from build123d import *

# Parameters (mm, degrees)
CROQUIS1_W                   = 75
CROQUIS1_H                   = 55
SALIENTE_EXTRUIR1_DEPTH      = 1.5
REDONDEO1_R                  = 3
TALADRO_DE_MARGEN_PARA_M31_D = 3.2
CROQUIS4_W                   = 14.87
CROQUIS4_H                   = 18.75
SALIENTE_EXTRUIR2_DEPTH      = 15.86
CROQUIS5_W                   = 30.45
CROQUIS5_H                   = 6.67
SALIENTE_EXTRUIR3_DEPTH      = 9.67
CROQUIS6_W                   = 15.19
CROQUIS6_H                   = 2.5
SALIENTE_EXTRUIR4_DEPTH      = 2.39
CROQUIS7_W                   = 0.67
CROQUIS7_H                   = 0.67
SALIENTE_EXTRUIR5_DEPTH      = 5.8


with BuildPart() as part:
    # Croquis1 → Saliente-Extruir1 (new body)
    with BuildSketch(Plane.XY):
        Rectangle(CROQUIS1_W, CROQUIS1_H)
    extrude(amount=SALIENTE_EXTRUIR1_DEPTH)

    # Redondeo1
    redondeo1_edges = [part.edges().sort_by_distance(p)[0] for p in [
        (-37.5, 27.5, 0.75),
        (37.5, 27.5, 0.75),
        (37.5, -27.5, 0.75),
        (-37.5, -27.5, 0.75),
    ]]
    fillet(redondeo1_edges, radius=REDONDEO1_R)

    # Taladro de margen para M31 (through all)
    with Locations(Plane.XY.offset(1.5)):
        with Locations((-34, 24), (-34, -24), (34, 24), (34, -24)):
            Hole(TALADRO_DE_MARGEN_PARA_M31_D / 2)

    # Croquis4 → Saliente-Extruir2 (add)
    with BuildSketch(Plane.XY.offset(1.5)):
        with Locations((-26.065, 4.905)):
            Rectangle(CROQUIS4_W, CROQUIS4_H)
        with Locations((-8.985, 4.905)):
            Rectangle(CROQUIS4_W, CROQUIS4_H)
        with Locations((8.985, 4.905)):
            Rectangle(CROQUIS4_W, CROQUIS4_H)
        with Locations((26.065, 4.905)):
            Rectangle(CROQUIS4_W, CROQUIS4_H)
    extrude(amount=SALIENTE_EXTRUIR2_DEPTH)

    # Croquis5 → Saliente-Extruir3 (add)
    with BuildSketch(Plane.XY.offset(1.5)):
        with Locations((-16.735, 19.265)):
            Rectangle(CROQUIS5_W, CROQUIS5_H)
        with Locations((16.735, 19.265)):
            Rectangle(CROQUIS5_W, CROQUIS5_H)
    extrude(amount=SALIENTE_EXTRUIR3_DEPTH)

    # Croquis6 → Saliente-Extruir4 (add)
    with BuildSketch(Plane.XY.offset(1.5)):
        with Locations((22.865, -22.54)):
            Rectangle(CROQUIS6_W, CROQUIS6_H)
    extrude(amount=SALIENTE_EXTRUIR4_DEPTH)

    # Croquis7 → Saliente-Extruir5 (add)
    with BuildSketch(Plane.XY.offset(3.89)):
        with Locations((16.465, -22.54)):
            Rectangle(CROQUIS7_W, CROQUIS7_H)
        with Locations((19.025, -22.54)):
            Rectangle(CROQUIS7_W, CROQUIS7_H)
        with Locations((21.585, -22.54)):
            Rectangle(CROQUIS7_W, CROQUIS7_H)
        with Locations((24.145, -22.54)):
            Rectangle(CROQUIS7_W, CROQUIS7_H)
        with Locations((26.705, -22.54)):
            Rectangle(CROQUIS7_W, CROQUIS7_H)
        with Locations((29.265, -22.54)):
            Rectangle(CROQUIS7_W, CROQUIS7_H)
    extrude(amount=SALIENTE_EXTRUIR5_DEPTH)


solid = part.part
CAD build for the part. Positions are in the model's coordinates, mm. A direction names the side the tool comes from. Round coordinates to 2 decimals unless told otherwise and drop trailing zeros. Write each loop counter-clockwise with the first axis right and the second up, starting at its lowest first coordinate (ties: lowest second). Pieces come first, ordered by that corner, then holes.
(1) 3-axis set-ups, long thin cutter, end or side, ignore diameter. For faces 4 (the face through (30.46, -23, 3)), 5 (the face through (-9, 14.28, 9)), 6 (the face through (33.5, 5, 9)), 7 (the face through (-1.51, 19, 6)), 8 (the face through (17, 22.6, 6)): which of +Z, -Z, +X, -X, +Y, -Y reach the whole face in a straight line?
(2) Mould opens along Y. For faces 1 (the face through (-26, 5, 17.36)), 2 (the face through (36.6, -26.64, 0.76)), 3 (the face through (-17, 15.93, 6)) say: pulls with the +Y half, pulls with the -Y half, needs draft (parallel to the pull), parting line crosses it, or undercut.
(3) Slice it at B-B, the plane z = 3. Write the cut outline in (x, y), and give its area (3 significant figures).
(4) Slice it at C-C, the plane y = 17. Write the cut outline in (x, z).
(5) Probe line 1 along Y through (x, z) = (34, 0.45); line 2 along X through (y, z) = (13, 8.75); line 3 along Y through (x, z) = (-5.5, 10.75). List the from-to ranges inside material, lowest first.
(6) Slice it at D-D, the plane x = -10. Write the cut outline in (y, z).
(7) Drop flat-ended pins along their axis: P1, Ø10, axis at y = 11.5, z = 7.5, coming from the +X side; P2, Ø4, axis at x = 20, z = 14.5, coming from the +Y side; P3, Ø7.5, axis at x = -25.5, z = 8, coming from the +Y side. Give the stop position or say it passes through.
(8) Slice it at A-A, the plane z = 15. Write the cut outline in (x, y), and give its area (3 significant figures).
From the geometry:
1. face 4: +Z, +X, -Y
1. face 5: +Z, +X, -X
1. face 6: +Z, +X, +Y, -Y
1. face 7: +Z, +Y, -Y
1. face 8: +Z, +X, -X, +Y
2. face 1: needs draft
2. face 2: pulls with the -Y half
2. face 3: undercut
3. outline: (-33.5, -4.47) - (-18.63, -4.47) - (-18.63, 14.28) - (-33.5, 14.28) - close; (-31.96, 15.93) - (-1.51, 15.93) - (-1.51, 22.6) - (-31.96, 22.6) - close; (-16.42, -4.47) - (-1.55, -4.47) - (-1.55, 14.28) - (-16.42, 14.28) - close; (1.51, 15.93) - (31.96, 15.93) - (31.96, 22.6) - (1.51, 22.6) - close; (1.55, -4.47) - (16.42, -4.47) - (16.42, 14.28) - (1.55, 14.28) - close; (15.27, -23.79) - (30.46, -23.79) - (30.46, -21.29) - (15.27, -21.29) - close; (18.63, -4.47) - (33.5, -4.47) - (33.5, 14.28) - (18.63, 14.28) - close
3. area: 1,560 mm2
4. outline: (-37.5, 0) - (37.5, 0) - (37.5, 1.5) - (31.96, 1.5) - (31.96, 11.17) - (1.51, 11.17) - (1.51, 1.5) - (-1.51, 1.5) - (-1.51, 11.17) - (-31.96, 11.17) - (-31.96, 1.5) - (-37.5, 1.5) - close
5. line 1: y = -27.5 to -25.6, -22.4 to 22.4, 25.6 to 27.5
5. line 2: x = -33.5 to -18.63, -16.42 to -1.55, 1.55 to 16.42, 18.63 to 33.5
5. line 3: y = -4.47 to 14.28, 15.93 to 22.6
6. outline: (-27.5, 0) - (27.5, 0) - (27.5, 1.5) - (22.6, 1.5) - (22.6, 11.17) - (15.93, 11.17) - (15.93, 1.5) - (14.28, 1.5) - (14.28, 17.36) - (-4.47, 17.36) - (-4.47, 1.5) - (-27.5, 1.5) - close
7. P1: stops at x = 33.5
7. P2: stops at y = 14.28
7. P3: stops at y = 22.6
8. outline: (-33.5, -4.47) - (-18.63, -4.47) - (-18.63, 14.28) - (-33.5, 14.28) - close; (-16.42, -4.47) - (-1.55, -4.47) - (-1.55, 14.28) - (-16.42, 14.28) - close; (1.55, -4.47) - (16.42, -4.47) - (16.42, 14.28) - (1.55, 14.28) - close; (18.63, -4.47) - (33.5, -4.47) - (33.5, 14.28) - (18.63, 14.28) - close
8. area: 1,120 mm2
